```python
from build123d import *

# Parameters (mm, degrees)
AUFSATZ_LINEAR_AUSTRAGEN1_DEPTH = 5
SKIZZE2_R                       = 2
AUFSATZ_LINEAR_AUSTRAGEN2_DEPTH = 5
SKIZZE3_R                       = 2.5
SCHNITT_LINEAR_AUSTRAGEN1_DEPTH = 31


with BuildPart() as part:
    # Skizze1 → Aufsatz-Linear austragen1 (new body)
    with BuildSketch(Plane(origin=(0, 0, 0), x_dir=(1, 0, 0), z_dir=(0, 1, 0))):
        with BuildLine():
            ThreePointArc((10, 0), (0, 10), (-10, 0))
            Line((-10, 0), (10, 0))
        make_face()
        with BuildLine():
            Line((10, 0), (-10, 0))
            ThreePointArc((-10, 0), (0, -10), (10, 0))
        make_face()
        with BuildLine():
            ThreePointArc((10, 0), (0, 10), (-10, 0))
            Line((-10, 0), (10, 0))
        make_face()
        with BuildLine():
            Line((10, 0), (-10, 0))
            ThreePointArc((-10, 0), (0, -10), (10, 0))
        make_face()
        with BuildLine():
            ThreePointArc((10, 0), (0, -10), (-10, 0))
            Line((-10, 0), (-10, -20))
            Line((-10, -20), (10, -20))
            Line((10, -20), (10, 0))
        make_face()
    extrude(amount=AUFSATZ_LINEAR_AUSTRAGEN1_DEPTH)

    # Skizze2 → Aufsatz-Linear austragen2 (add)
    with BuildSketch(Plane(origin=(0, 5, 0), x_dir=(1, 0, 0), z_dir=(0, 1, 0))):
        with Locations(Location((0, 0, 0), (0, 0, 270))):
            Circle(SKIZZE2_R)
        with BuildLine():
            Line((-10, -20), (10, -20))
            Line((10, -20), (10, 0))
            ThreePointArc((10, 0), (0, -10), (-10, 0))
            Line((-10, 0), (-10, -20))
        make_face()
    extrude(amount=AUFSATZ_LINEAR_AUSTRAGEN2_DEPTH)

    # Skizze3 → Schnitt-Linear austragen1 (cut, through all)
    with BuildSketch(Plane(origin=(10, 0, 0), x_dir=(0, 0, -1), z_dir=(1, 0, 0))):
        with Locations((-15, 5)):
            Circle(SKIZZE3_R)
    extrude(amount=-SCHNITT_LINEAR_AUSTRAGEN1_DEPTH, mode=Mode.SUBTRACT)


solid = part.part
```
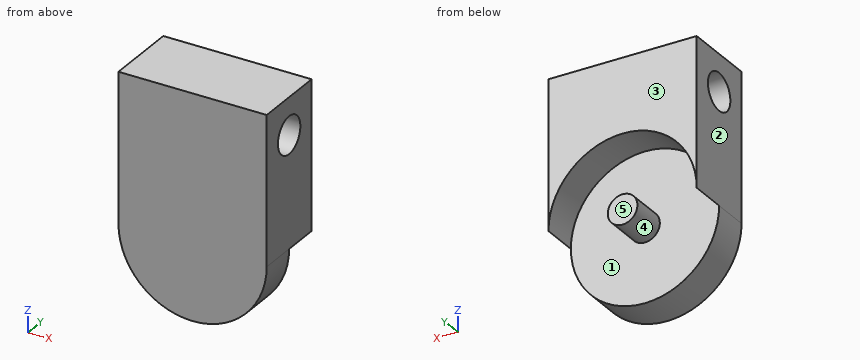
CAD build for the part. Positions are in the model's coordinates, mm. Face numbers are marked on the shaded views. A direction names the side the tool comes from. Coordinates: 2 decimals unless noted, no trailing zeros. Write each loop counter-clockwise with the first axis right and the second up, starting at its lowest first coordinate (ties: lowest second). Pieces come first, ordered by that corner, then holes. Notation, with made-up numbers: (59.5, -40) -> (102.5, -40) arc R6 cw to (102.5, -31) -> close; hole circle Ø5 at (-29, -33). An arc over 180 degrees is marked (long way). Return JSON: item names as keys, results as strings. Group by question number.
Q1. Pull direction X, two halves, no side cores. Call the marked faces 1, 2 and 3: released by +X, released by -X, zero draft, split by the parting line, or undercut.
Q2. Flat gauge pins, fed straight in: pin 1 (1 mm diameter, centred on y = 4, z = -2.5, fed in from +X); pin 2 (4.5 mm diameter, centred on y = 5, z = 15, fed in from +X). Where does each tip first touch, or does it go through?
Q3. Cut at B-B, the plane x = 0. Give the cut face in (y, z), then the cut area to 3 significant figures.
Q4. Which spindle directions (+Z, -Z, +X, -X, +Y, -Y) get a long thin tool onto all of the face, cutting with end or side? Do the marked faces 4 and 5. Say none if no direction does.
Q5. Drill centre lines: line 1 (Y direction, x = 2.5, z = 15); line 2 (Y direction, x = -5.75, z = 4.75); line 3 (Z direction, x = 0.5, y = 3.25). Where is each one in solid material? Low to high.
Q6. Cut at A-A, the plane z = 15. Give the cut face in (x, y).
Q7. Cut at D-D, the plane y = 3.25. Give the cut face in (x, z), then the cut area to 3 significant figures.
Q8. Cut at C-C, the plane y = 6.75. Give the cut face in (x, z), then the cut area to 3 significant figures.
Returned:
{
 "1": {"face 1": "undercut", "face 2": "released by -X", "face 3": "zero draft"},
 "2": {"pin 1": "stops at x = 9.8", "pin 2": "passes through"},
 "3": {"outline": "(0, -10) -> (5, -10) -> (5, -2) -> (10, -2) -> (10, 2) -> (5, 2) -> (5, 10) -> (10, 10) -> (10, 20) -> (0, 20) -> close; hole circle Ø5 at (5, 15)", "area": "200 mm2"},
 "4": {"face 4": "+Y", "face 5": "+Z, -Z, +X, -X, +Y"},
 "5": {"line 1": "y = 0 to 2.5, 7.5 to 10", "line 2": "y = 0 to 5", "line 3": "z = -9.99 to 13.21, 16.79 to 20"},
 "6": {"outline": "(-10, 0) -> (10, 0) -> (10, 2.5) -> (-10, 2.5) -> close; (-10, 7.5) -> (10, 7.5) -> (10, 10) -> (-10, 10) -> close"},
 "7": {"outline": "(-10, 0) arc R10 ccw to (10, 0) -> (10, 13.21) -> (-10, 13.21) -> close; (-10, 16.79) -> (10, 16.79) -> (10, 20) -> (-10, 20) -> close", "area": "486 mm2"},
 "8": {"outline": "(-10, 0) arc R10 cw to (10, 0) -> (10, 13.21) -> (-10, 13.21) -> close; (-10, 16.79) -> (10, 16.79) -> (10, 20) -> (-10, 20) -> close; circle Ø4 at (0, 0)", "area": "184 mm2"}
}
